Autodesk Inventor part; units mm, degrees
ref_plane "Work Plane1" through (0, 3.175, 15) normal (0, 1, 0) x (1, 0, 0)
ref_plane "Work Plane3" through (11.5, -12, 0) normal (1, 0, 0) x (0, 0, -1)
ref_plane "Work Plane4" through (11.5, -12, 0) normal (1, 0, 0) x (0, 0, -1)
sketch "Sketch1" plane through (0, 0, 0) normal (0, 0, 1) x (1, 0, 0)
  line L0 (-4.3, 0) -> (27.3, 0)
  line L1 (27.5, -0.2) -> (27.5, -5.5)
  line L2 (-4.3, -12) -> (27.3, -12)
  line L3 (27.5, -6.5) -> (27.5, -11.8)
  line L4 (-4.5, -0.2) -> (-4.5, -5.5)
  line L5 (-4.5, -6.5) -> (-4.5, -11.8)
  line L6 (-4.5, 0) -> (-1.071, 0)
  line L7 (-1.071, 0) -> (-1.071, -12)
  line L8 (-1.071, -12) -> (-4.5, -12)
  line L9 (-4.5, -12) -> (-4.5, 0)
  arc A0 (-3.366, -6.5) -> (-3.366, -5.5) centre (-2.5, -6) ccw
  circle A1 centre (-2.5, -6) radius 1
  line L10 (27.5, -12) -> (24.071, -12)
  line L11 (24.071, -12) -> (24.071, 0)
  line L12 (24.071, 0) -> (27.5, 0)
  line L13 (27.5, 0) -> (27.5, -12)
  arc A2 (26.366, -5.5) -> (26.366, -6.5) centre (25.5, -6) ccw
  circle A3 centre (25.5, -6) radius 1
  line L14 (-1.071, 0) -> (-4.5, 0)
  line L15 (-4.5, 0) -> (-4.5, 1.905)
  line L16 (-4.5, 1.905) -> (-1.071, 1.905)
  line L17 (-1.071, 1.905) -> (-1.071, 0)
  line L18 (11.5, 0) -> (11.5, -12) construction
  line L19 (27.5, 0) -> (24.071, 0)
  line L20 (24.071, 0) -> (27.5, 0)
  line L21 (27.5, 0) -> (27.5, 1.905)
  line L22 (27.5, 1.905) -> (24.071, 1.905)
  line L23 (24.071, 1.905) -> (24.071, 0)
  line L24 (-4.5, 1.905) -> (-1.071, 1.905)
  line L25 (-1.071, 1.905) -> (-1.071, 5.08)
  line L26 (-1.071, 5.08) -> (-4.5, 5.08)
  line L27 (-4.5, 5.08) -> (-4.5, 1.905)
  line L28 (24.071, 1.905) -> (27.5, 1.905)
  line L29 (27.5, 1.905) -> (27.5, 5.08)
  line L30 (27.5, 5.08) -> (24.071, 5.08)
  line L31 (24.071, 5.08) -> (24.071, 1.905)
  point P0 (0, 0)
  dimension "d0" = 3.429
  dimension "d1" = 3.429
  dimension "d2" = 1.905
  dimension "d8" = 3.175
  dimension "d9" = 3.175
extrude "Extrusion1" add sketch "Sketch1" along normal blind 1.905 contours L6 L15 L16 L17 L0 | L0 L7 L2 L8 L9 L5 L4 L6 | L23 L22 L21 L12 L0 | L0 L12 L13 L1 L3 L10 L2 L11 | L16 L27 L26 L25 | L31 L30 L29 L22
ref_plane "Work Plane1" through (0, 3.175, 15) normal (0, 1, 0) x (1, 0, 0)
sketch "Sketch2" plane through (0, 3.175, 15) normal (0, 1, 0) x (1, 0, 0)
  line L0 (-1.071, 15) -> (-4.5, 15)
  line L1 (-4.5, 15) -> (-4.5, 13.095)
  line L2 (-1.071, 13.095) -> (-4.5, 13.095)
  line L3 (-1.071, 15) -> (-1.071, 13.095)
  line L4 (27.5, 15) -> (24.071, 15)
  line L5 (24.071, 15) -> (24.071, 13.095)
  line L6 (27.5, 13.095) -> (24.071, 13.095)
  line L7 (27.5, 15) -> (27.5, 13.095)
  line L8 (22.8, 0) -> (0.2, 0)
  line L9 (-4.5, 13.095) -> (27.5, 13.095)
  line L10 (27.5, -3.175) -> (-4.5, -3.175)
  line L11 (-4.5, 11.19) -> (-1.071, 11.19)
  line L12 (-1.071, 11.19) -> (-1.071, 0)
  line L13 (-1.071, 0) -> (-4.5, 0)
  line L14 (27.5, 0) -> (24.071, 0)
  line L15 (24.071, 0) -> (24.071, 11.19)
  line L16 (24.071, 11.19) -> (27.5, 11.19)
  line L17 (23, 15) -> (23, 5)
  line L18 (0, 5) -> (0, 15)
  line L19 (-1.071, 15) -> (-1.071, 13.095)
  line L20 (24.071, 15) -> (24.071, 13.095)
  arc A0 (-1.071, 7.761) -> (-4.5, 11.19) centre (-4.5, 7.761) ccw
  arc A1 (-4.5, 0) -> (-1.071, 3.429) centre (-4.5, 3.429) ccw
  arc A2 (27.5, 11.19) -> (24.071, 7.761) centre (27.5, 7.761) ccw
  arc A3 (24.071, 3.429) -> (27.5, 0) centre (27.5, 3.429) ccw
  line L21 (-4.5, -3.175) -> (-4.5, 0)
  line L22 (-4.5, 11.19) -> (-4.5, 13.095)
  line L23 (27.5, 13.095) -> (27.5, 11.19)
  line L24 (27.5, 0) -> (27.5, -3.175)
  line L25 (27.5, 11.19) -> (27.5, 0)
  line L26 (-4.5, 11.19) -> (-4.5, 0)
  dimension "d5" = 3.175
  dimension "d13" = 1.905
extrude "Extrusion2" add sketch "Sketch2" along normal blind 1.905 contours L9 L6 L23 L16 L15 L14 L24 L10 L21 L13 L12 L11 L22 L2 | L11 L12 A0 | A0 L12 A1 L26 | A1 L12 L13 | A2 L15 L16 | L25 A3 L15 A2 | L14 L15 A3
sketch "Sketch6" plane through (0, 3.175, 15) normal (0, -1, 0) x (1, 0, 0)
  line L0 (0.2, 0) -> (22.8, 0)
  line L1 (-4.5, -15) -> (-4.5, 3.175)
  line L2 (27.5, 3.175) -> (-4.5, 3.175)
  line L3 (-4.5, 3.175) -> (-4.5, 1.27)
  line L4 (-4.5, 1.27) -> (27.5, 1.27)
  line L5 (27.5, 1.27) -> (27.5, 3.175)
  line L6 (27.5, 3.175) -> (27.5, -13.095)
  line L7 (-4.5, 3.175) -> (27.5, 3.175)
  point P0 (0, -15)
  dimension "d10" = 1.905
extrude "Extrusion3" add sketch "Sketch6" along normal up to surface (15.175 mm away)
sketch "Sketch7" plane through (-4.5, 5.08, 18.175) normal (0, 0, 1) x (1, 0, 0)
  line L0 (32, -17.08) -> (32, 0)
  line L1 (0, 0) -> (32, 0)
  line L2 (0, -17.08) -> (0, 0)
  line L3 (0, -17.08) -> (32, -17.08)
  line L4 (32, -17.08) -> (0, -17.08) construction
  line L5 (32, -17.08) -> (32, 0) construction
  circle A0 centre (10.5, -11.08) radius 1.5875
  circle A1 centre (10.5, -11.08) radius 3.75
  point P0 (4.5, -5.08)
  point P1 (31.8064, -17.08)
  point P2 (0.1936, -17.08)
  dimension "d15" = 3.175
sketch "Sketch8" plane through (24.071, 5.08, 0) normal (0, 1, 0) x (1, 0, 0)
  line L0 (3.429, 0) -> (3.429, -18.175)
  line L1 (3.429, 0) -> (0, 0)
  line L2 (0, 0) -> (0, -1.905)
  line L3 (0, -1.905) -> (-25.142, -1.905)
  line L4 (-25.142, 0) -> (-25.142, -1.905)
  line L5 (-25.142, 0) -> (-28.571, 0)
  line L6 (-28.571, 0) -> (-28.571, -18.175)
  line L7 (-28.571, -18.175) -> (3.429, -18.175)
  line L8 (-25.142, -7.239) -> (-25.142, -11.571) construction
  circle A0 centre (-18.071, -9.405) radius 1.5875
  line L9 (-21.821, 16.1332) -> (-14.321, 16.1332)
  line L10 (-18.071, 16.1332) -> (-18.071, -9.3987) construction
  line L11 (-25.142, -9.405) -> (0, -9.405) construction
  point P0 (-24.071, 0)
  dimension "d16" = 3.175
extrude "Extrusion4" cut sketch "Sketch8" against normal up to next contours A0
extrude "Extrusion5" cut sketch "Sketch7" against normal up to next contours A0
ref_plane "Work Plane3" through (11.5, -12, 0) normal (1, 0, 0) x (0, 0, -1)
mirror "Mirror1" about plane through (11.5, -12, 0) normal (1, 0, 0) of "Extrusion5"
mirror "Mirror2" about plane through (11.5, -12, 0) normal (1, 0, 0) of "Extrusion4"
sketch "Sketch9" plane through (27.5, 3.175, 16.27) normal (0, 0, -1) x (-1, 0, 0)
  circle A0 centre (2, -9.175) radius 1
  line L0 (3.429, 1.905) -> (3.429, -15.175)
  line L1 (0, 1.905) -> (3.429, 1.905)
  line L2 (0, -15.175) -> (0, 1.905)
  line L3 (3.429, -15.175) -> (0, -15.175)
  circle A1 centre (30, -9.175) radius 1
  line L4 (28.571, -15.175) -> (28.571, 1.905)
  line L5 (32, -15.175) -> (28.571, -15.175)
  line L6 (32, 1.905) -> (32, -15.175)
  line L7 (28.571, 1.905) -> (32, 1.905)
  line L8 (0, -15.175) -> (3.429, -15.175)
  line L9 (3.429, -15.175) -> (3.429, -11.365)
  line L10 (3.429, -11.365) -> (0, -11.365)
  line L11 (0, -11.365) -> (0, -15.175)
  line L12 (0, 0) -> (32, 0)
  line L13 (0, 0) -> (3.429, 0)
  line L14 (3.429, 0) -> (3.429, -7.62)
  line L15 (3.429, -7.62) -> (0, -7.62)
  line L16 (0, -7.62) -> (0, 0)
  point P0 (27.5, -3.175)
  dimension "d21" = 7.62
  dimension "d22" = 3.81
extrude "Extrusion6" add sketch "Sketch9" along normal up to next contours L0 L15 L2 L12 | L0 L3 L2 L10
ref_plane "Work Plane4" through (11.5, -12, 0) normal (1, 0, 0) x (0, 0, -1)
mirror "Mirror3" about plane through (11.5, -12, 0) normal (1, 0, 0) of "Extrusion6"
sketch "Sketch10" plane through (24.071, 3.175, 1.905) normal (0, 0, -1) x (-1, 0, 0)
  line L0 (25.142, 0) -> (25.142, 1.905)
  line L1 (0, 1.905) -> (25.142, 1.905)
  line L2 (0, 1.905) -> (0, 0)
  line L3 (0, 0) -> (25.142, 0)
  point P0 (24.071, -3.175)
extrude "Extrusion7" add sketch "Sketch10" along normal up to surface (1.905 mm away)
sketch "Sketch11" plane through (24.071, 3.175, 16.27) normal (0, 0, -1) x (-1, 0, 0)
  line L0 (25.142, -15.175) -> (25.142, -11.365)
  line L1 (25.142, -11.365) -> (28.571, -11.365)
  line L2 (28.571, -7.62) -> (28.571, -11.365)
  line L3 (28.571, -7.62) -> (25.142, -7.62)
  line L4 (25.142, -7.62) -> (25.142, 0)
  line L5 (0, 0) -> (25.142, 0)
  line L6 (0, 0) -> (0, -7.62)
  line L7 (0, -7.62) -> (-3.429, -7.62)
  line L8 (-3.429, -7.62) -> (-3.429, -11.365)
  line L9 (-3.429, -11.365) -> (0, -11.365)
  line L10 (0, -11.365) -> (0, -15.175)
  line L11 (0, -15.175) -> (25.142, -15.175)
  circle A0 centre (7.071, -9.175) radius 1.5875
  circle A1 centre (18.071, -9.175) radius 1.5875
  line L12 (0, -7.62) -> (0, -11.365)
  point P0 (24.071, -3.175)
extrude "Extrusion8" add sketch "Sketch11" along normal blind 5.08 contours L9 L8 L7 L12
fillet "Fillet2" radius 1.8542 2 edges at (25.7855, -4.445, 11.19) (25.7855, -8.19, 11.19)
mirror "Mirror4" about plane through (11.5, -12, 0) normal (1, 0, 0) of "Extrusion8"
mirror "Mirror5" about plane through (11.5, -12, 0) normal (1, 0, 0) of "Fillet2"
properties part number "Servo_vice_real"
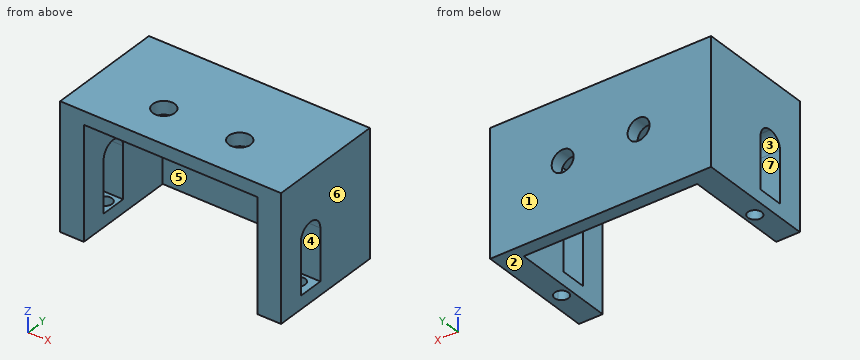
The model under review builds one solid part; all positions refer to its coordinate system, in mm. Face numbers are marked on the shaded views. A direction names the side the tool comes from. Round coordinates to 2 decimals unless told otherwise and drop trailing zeros. Order: outer loops, then holes, each group sorted by start corner. A loop starts at its lowest first (then second) coordinate and runs counter-clockwise, first axis right, second up. Notation, with made-up numbers: (19, 46.5) -> (78, 46.5) arc R15 ccw to (78, 73.5) -> close; hole circle Ø9 at (-35.5, 56.5). An arc over 180 degrees is marked (long way). Use a Markdown table: item, result.
Q1. Tool access review of the marked faces 5, 6 and 7: name each direction out of +Z, -Z, +X, -X, +Y, -Y from which nothing blocks a thin tool from reaching the whole face with its end or side.
Values:
| item | result |
|---|---|
| face 5 | -Z, -Y |
| face 6 | +Z, -Z, +X, +Y, -Y |
| face 7 | +X, -X |
Q2. We need section D-D on x = -2.5. Write out the cut boundary in (y, z) (3 decimals), then the cut area to 3 significant figures.
Values:
| item | result |
|---|---|
| outline | (-12, 0) -> (-7, 0) -> (-7, 1.905) -> (-8.19, 1.905) -> (-8.19, 9.336) arc R1.854 cw to (-6.336, 11.19) -> (-6.299, 11.19) arc R1.854 cw to (-4.445, 9.336) -> (-4.445, 1.905) -> (-5, 1.905) -> (-5, 0) -> (5.08, 0) -> (5.08, 18.175) -> (-12, 18.175) -> close |
| area | 273 mm^2 |
Q3. We need section B-B on y = -1.5. Write out the cut boundary in (x, z) (3 decimals), then the cut area to 3 significant figures.
Values:
| item | result |
|---|---|
| outline | (-4.5, 0) -> (-1.071, 0) -> (-1.071, 16.27) -> (24.071, 16.27) -> (24.071, 0) -> (27.5, 0) -> (27.5, 18.175) -> (-4.5, 18.175) -> close |
| area | 173 mm^2 |
Q4. For line 1 (Y direction, x = 6, z = 16.7); line 2 (Y direction, x = -2.5, z = 1.2); line 3 (X direction, y = -8.5, z = 1.5), list the stretches that pass through material, from the lowest coordinate up.
Values:
| item | result |
|---|---|
| line 1 | y = -12 to -7.59, -4.41 to 5.08 |
| line 2 | y = -12 to -7, -5 to 5.08 |
| line 3 | x = -4.5 to -1.07, 24.07 to 27.5 |
Q5. We need section A-A on x = 17. Write out the cut boundary in (y, z) (1 decimal), then the cut area to 3 significant figures.
Values:
| item | result |
|---|---|
| outline | (-12, 16.3) -> (-7.6, 16.3) -> (-7.6, 18.2) -> (-12, 18.2) -> close; (-4.4, 16.3) -> (3.2, 16.3) -> (3.2, 11) -> (5.1, 11) -> (5.1, 18.2) -> (-4.4, 18.2) -> close; (3.2, 0) -> (5.1, 0) -> (5.1, 7.8) -> (3.2, 7.8) -> close |
| area | 51.4 mm^2 |
Q6. Mouldability with a two-part tool opening along Y and no side actions: class the marked faces 1, 2, 3 and 4 as +Y half, -Y half, draft (parallel to the pull), parting line (faces both ways), or undercut.
Values:
| item | result |
|---|---|
| face 1 | +Y half |
| face 2 | draft |
| face 3 | undercut |
| face 4 | undercut |
Q7. Clearance check with flat-ended pins moving along their axes: P1, Ø3, axis at x = 17, z = 9.405, coming from the +Y side; P2, Ø7.5, axis at x = 11.5, y = -2, coming from the -Z side. State where each tip first meets the part, or that it passes through.
Values:
| item | result |
|---|---|
| P1 | passes through |
| P2 | stops at z = 16.27 |
Q8. We need section C-C on z = 12.5. Write out the cut boundary in (x, y) (3 decimals), then the cut area to 3 significant figures.
Values:
| item | result |
|---|---|
| outline | (-4.5, -12) -> (-1.071, -12) -> (-1.071, 3.175) -> (24.071, 3.175) -> (24.071, -12) -> (27.5, -12) -> (27.5, 5.08) -> (-4.5, 5.08) -> close |
| area | 165 mm^2 |
